Autodesk Inventor part; units mm, degrees
ref_plane "YZ Plane" through (0, 0, 0) normal (1, 0, 0) x (0, 1, 0)
ref_plane "XZ Plane" through (0, 0, 0) normal (0, 1, 0) x (-1, 0, 0)
ref_plane "XY Plane" through (0, 0, 0) normal (0, 0, 1) x (1, 0, 0)
sketch "Sketch1" plane through (0, 0, 0) normal (0, 1, 0) x (-1, 0, 0)
  line L0 (-2.9393, 4) -> (2.9393, 4)
  line L1 (4, 2.9393) -> (4, -2.9393)
  line L2 (2.9393, -4) -> (-2.9393, -4)
  line L3 (-4, -2.9393) -> (-4, 2.9393)
  circle A0 centre (0, 0) radius 2.15
  line L4 (-2.9393, 4) -> (-6.75, 7.8107)
  line L5 (-7.8107, 6.75) -> (-4, 2.9393)
  line L6 (4, -2.9393) -> (7.8107, -6.75)
  line L7 (-10, 10) -> (-2.5, 10)
  line L8 (2.5, 10) -> (10, 10)
  line L9 (10, -10) -> (2.5, -10)
  line L10 (-2.5, -10) -> (-10, -10)
  line L11 (10, 10) -> (10, 2.5)
  line L12 (10, -2.5) -> (10, -10)
  line L13 (-10, -10) -> (-10, -2.5)
  line L14 (-10, 2.5) -> (-10, 10)
  line L15 (-8.5, 2.5) -> (-8.5, 6.75)
  line L16 (-6.75, 8.5) -> (-2.5, 8.5)
  line L17 (2.5, 10) -> (2.5, 8.5)
  line L18 (10, 2.5) -> (8.5, 2.5)
  line L19 (10, -2.5) -> (8.5, -2.5)
  line L20 (2.5, -8.5) -> (2.5, -10)
  line L21 (-2.5, -8.5) -> (-2.5, -10)
  line L22 (-8.5, -2.5) -> (-10, -2.5)
  line L23 (-8.5, 2.5) -> (-10, 2.5)
  line L24 (-2.5, 10) -> (-2.5, 8.5)
  line L25 (-7.8107, 6.75) -> (-8.5, 6.75)
  line L26 (-6.75, 8.5) -> (-6.75, 7.8107)
  line L27 (6.75, 8.5) -> (6.75, 7.8107)
  line L28 (8.5, 6.75) -> (7.8107, 6.75)
  line L29 (8.5, 6.75) -> (8.5, 2.5)
  line L30 (2.5, 8.5) -> (6.75, 8.5)
  line L31 (6.75, 7.8107) -> (2.9393, 4)
  line L32 (7.8107, 6.75) -> (4, 2.9393)
  line L33 (2.9393, -4) -> (6.75, -7.8107)
  line L34 (8.5, -2.5) -> (8.5, -6.75)
  line L35 (6.75, -8.5) -> (2.5, -8.5)
  line L36 (8.5, -6.75) -> (7.8107, -6.75)
  line L37 (6.75, -7.8107) -> (6.75, -8.5)
  line L38 (-2.5, -8.5) -> (-6.75, -8.5)
  line L39 (-2.9393, -4) -> (-6.75, -7.8107)
  line L40 (-8.5, -6.75) -> (-8.5, -2.5)
  line L41 (-4, -2.9393) -> (-7.8107, -6.75)
  line L42 (-6.75, -7.8107) -> (-6.75, -8.5)
  line L43 (-7.8107, -6.75) -> (-8.5, -6.75)
  dimension "d0" = 20
  dimension "d1" = 20
  dimension "d26" = 1.5
  dimension "d27" = 1.5
  dimension "d32" = 7.5
  dimension "d33" = 5
  dimension "d34" = 7.5
  dimension "d35" = 7.5
  dimension "d40" = 6
  dimension "d41" = 13.5
extrude "Extrusion1" add sketch "Sketch1" along normal blind 250
chamfer "Chamfer1" distance 0.5 angle 45 12 edges at (-10, 125, 2.5) (-10, 125, -2.5) (-2.5, 125, 10) (2.5, 125, 10) (10, 125, 2.5) (10, 125, -2.5) (2.5, 125, -10) (-2.5, 125, -10) (-10, 125, 10) (-10, 125, -10) (10, 125, -10) (10, 125, 10)
properties part number "2020 Extrusion 250mm" material "Aluminum 6061"
Geometry: final body of the model. Coordinates: model frame, mm. A direction names the side the tool comes from. Coordinates: 2 decimals unless noted, no trailing zeros. Order: outer loops, then holes, each group sorted by start corner. A loop starts at its lowest first (then second) coordinate and runs counter-clockwise, first axis right, second up.
1) Ray query, probe 1 along Z at (x, y) = (0, 82.5); probe 2 along Z at (x, y) = (-6, 27); probe 3 along Z at (x, y) = (1, 36). Return the intervals inside material, ascending.
Result sheet:
probe 1: z = -4 to -2.15, 2.15 to 4
probe 2: z = -10 to -8.5, -7.06 to -4.94, 4.94 to 7.06, 8.5 to 10
probe 3: z = -4 to -1.9, 1.9 to 4
2) Draft query along Z for faces 1 (the flat face through (-5.93, 123.25, 4.87)), 2 (the flat face through (-8.5, 123, -5)), 3 (the flat face through (6, 123, -10)), 4 (the flat face through (10, 123, -6)). Return one class per face: released by +Z, released by -Z, zero draft, split by the parting line, or undercut.
Result sheet:
face 1: undercut
face 2: undercut
face 3: released by -Z
face 4: zero draft
3) First-contact query: P1, Ø2, axis at x = 0.5, y = 52.5, coming from the -Z side; P2, Ø3, axis at y = 180, z = -0.5, coming from the -X side. Flat tips, straight axial feed; report the tip coordinate or a pass-through.
Result sheet:
P1: stops at z = -4
P2: stops at x = -4
4) Section A-A (x = 0). Return loops of the section in (y, z), then the cut area to 3 significant figures.
Result sheet:
outline: (0, -4) - (250, -4) - (250, -2.15) - (0, -2.15) - close; (0, 2.15) - (250, 2.15) - (250, 4) - (0, 4) - close
area: 925 mm2
5) Set-up query: faces 5 (the flat face through (5.88, 123.25, -4.82)), 6 (the flat face through (-6, 123, -10)). Return all of +Z, -Z, +X, -X, +Y, -Y with unobstructed straight access to the full face (end or side cutting, diameter ignored); none if empty.
Result sheet:
face 5: +Y, -Y
face 6: -Z, +X, -X, +Y, -Y
6) Section B-B (z = 0). Return loops of the section in (x, y), then the cut area to 3 significant figures.
Result sheet:
outline: (-4, 0) - (-2.15, 0) - (-2.15, 250) - (-4, 250) - close; (2.15, 0) - (4, 0) - (4, 250) - (2.15, 250) - close
area: 925 mm2
